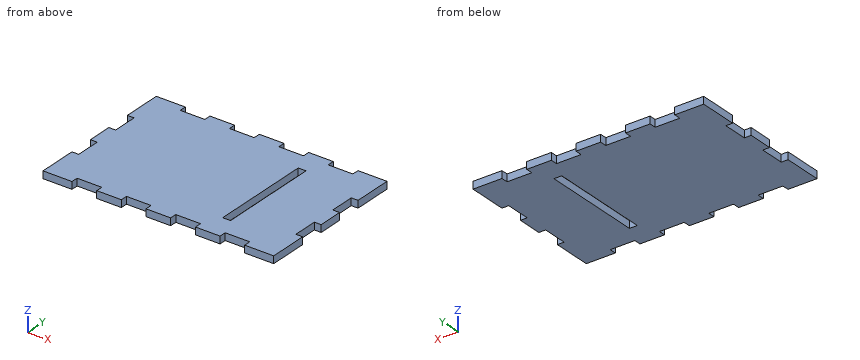
```python
from build123d import *

# Parameters (mm, degrees)
BOSS_EXTRUDE1_DEPTH = 6.35
SKETCH4_W           = 6.888524177
SKETCH4_H           = 88.9
CUT_EXTRUDE1_DEPTH  = 6.35


with BuildPart() as part:
    # Sketch3 → Boss-Extrude1 (new body)
    with BuildSketch(Plane.XY):
        Polygon((0, 77.53985), (0, 55.81015), (5.9944, 55.81015), (5.9944, 34.08045), (0, 34.08045), (0, 12.35075), (0, 0), (25.54605, 0), (25.54605, 5.9944), (47.27575, 5.9944), (47.27575, 0), (69.00545, 0), (69.00545, 5.9944), (90.73515, 5.9944), (90.73515, 0), (112.46485, 0), (112.46485, 5.9944), (134.19455, 5.9944), (134.19455, 0), (155.92425, 0), (155.92425, 5.9944), (177.65395, 5.9944), (177.65395, 0), (203.2, 0), (203.2, 34.08045), (197.2056, 34.08045), (197.2056, 55.81015), (203.2, 55.81015), (203.2, 77.53985), (197.2056, 77.53985), (197.2056, 99.26955), (203.2, 99.26955), (203.2, 120.99925), (203.2, 133.35), (177.65395, 133.35), (177.65395, 127.3556), (155.92425, 127.3556), (155.92425, 133.35), (134.19455, 133.35), (134.19455, 127.3556), (112.46485, 127.3556), (112.46485, 133.35), (90.73515, 133.35), (90.73515, 127.3556), (69.00545, 127.3556), (69.00545, 133.35), (47.27575, 133.35), (47.27575, 127.3556), (25.54605, 127.3556), (25.54605, 133.35), (0, 133.35), (0, 99.26955), (5.9944, 99.26955), (5.9944, 77.53985), align=None)
    extrude(amount=BOSS_EXTRUDE1_DEPTH)

    # Sketch4 → Cut-Extrude1 (cut)
    with BuildSketch(Plane.XY.offset(6.35)):
        with Locations((145.073671488, 66.675)):
            Rectangle(SKETCH4_W, SKETCH4_H)
    extrude(amount=-CUT_EXTRUDE1_DEPTH, mode=Mode.SUBTRACT)


solid = part.part
```
Geometry: final body of the model. Coordinates: model frame, mm. Round coordinates to 2 decimals unless told otherwise and drop trailing zeros. Write each loop counter-clockwise with the first axis right and the second up, starting at its lowest first coordinate (ties: lowest second). Pieces come first, ordered by that corner, then holes. Notation, with made-up numbers: (25.25, -34.75) -> (47.25, -34.75) arc R15 cw to (47.25, -29.75) -> close; hole circle Ø5 at (-18, 63). An arc over 180 degrees is marked (long way). Return JSON: item names as keys, results as strings.
Q1. Section C-C on x = 166. Return the cut outline in (y, z), and give its area (3 significant figures).
From the geometry:
{"outline": "(5.99, 0) -> (127.36, 0) -> (127.36, 6.35) -> (5.99, 6.35) -> close", "area": "771 mm2"}
Q2. Section A-A on y = 81.5. Return the cut outline in (x, z).
From the geometry:
{"outline": "(5.99, 0) -> (141.63, 0) -> (141.63, 6.35) -> (5.99, 6.35) -> close; (148.52, 0) -> (197.21, 0) -> (197.21, 6.35) -> (148.52, 6.35) -> close"}
Q3. Section B-B on y = 59. Return the cut outline in (x, z).
From the geometry:
{"outline": "(0, 0) -> (141.63, 0) -> (141.63, 6.35) -> (0, 6.35) -> close; (148.52, 0) -> (203.2, 0) -> (203.2, 6.35) -> (148.52, 6.35) -> close"}
Q4. Ray query, line 1 (X direction, y = 91.5, z = 0.5); line 2 (X direction, y = 30, z = 5); line 3 (Y direction, x = 142, z = 1.25) (3 decimals). Return the intervals inside material, ascending.
From the geometry:
{"line 1": "5.99 to 141.63, 148.52 to 197.21", "line 2": "0 to 141.63, 148.52 to 203.2", "line 3": "0 to 22.225, 111.125 to 133.35"}
Q5. First-contact query: pin 1 Ø3 at (y, z) = (51.5, 3.5) entering from -X; pin 2 Ø2 at (x, z) = (133, 2) entering from -Y; pin 3 Ø2 at (x, z) = (69, 5.5) entering from -Y; pin 4 Ø3 at (y, z) = (88.5, 2.5) entering from +X. Flat tips, straight axial feed; report the tip coordinate or a pass-through.
From the geometry:
{"pin 1": "x = 5.99", "pin 2": "y = 5.99", "pin 3": "y = 0", "pin 4": "x = 197.21"}
